The model under review builds one solid part; all positions refer to its coordinate system, in mm. Face numbers are marked on the shaded views. A direction names the side the tool comes from. Coordinates: 2 decimals unless noted, no trailing zeros. Write each loop counter-clockwise with the first axis right and the second up, starting at its lowest first coordinate (ties: lowest second). Pieces come first, ordered by that corner, then holes. Notation, with made-up numbers: (68, -33) - (85, -33) arc R14 ccw to (85, -19) - close; hole circle Ø7 at (-32, 88.5). An arc over 180 degrees is marked (long way). Put each result on its own line as item: value. Start each with the question number.
Item 1: Consider section A-A on y = 0. Give the boundary of the cut face in (x, z) (3 decimals).
Item 2: Consider section D-D on x = 4.5. Give the boundary of the cut face in (y, z).
Item 3: For pin 1 (10 mm diameter, centred on y = -10.5, z = 47.5, fed in from -X); pin 2 (10 mm diameter, centred on x = -6.5, z = 52.5, fed in from +Y); pin 3 (5.5 mm diameter, centred on x = 0, y = 0, fed in from +Z); pin 4 (8 mm diameter, centred on x = 4.5, z = 56, fed in from -Y), all flat-tipped, find the tip position at first contact; note any pin that passes through.
Item 4: Machinability: for the marked faces 1 and 2, which of the approach directions +Z, -Z, +X, -X, +Y, -Y give a long, thin tool a straight path to every point of the face, cutting with its end or side? Answer none if there is none.
Item 5: Consider section C-C on z = 33.5. Give the boundary of the cut face in (x, y) (3 decimals).
Item 6: To check wall thickness, follow L1, parallel to Y at x = 0, z = 19 (3 decimals); L2, parallel to Z at x = 10, y = -4; L3, parallel to X at y = -1, z = 7. State the ranges of each line that lie inside material, in increasing order. Write a range as [from, to].
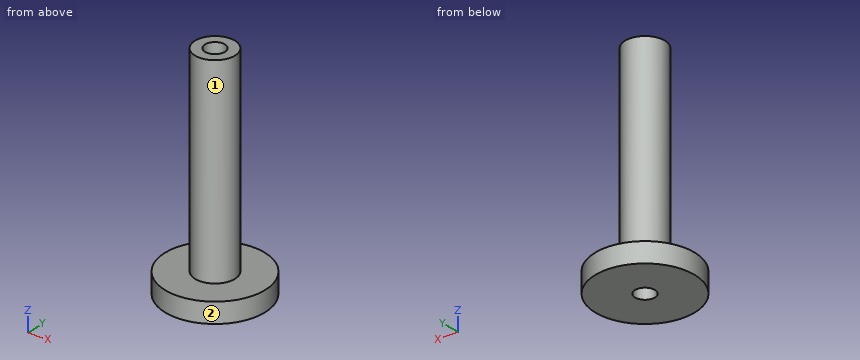
Autodesk Inventor part; units mm, degrees
ref_plane "YZ Plane" through (0, 0, 0) normal (1, 0, 0) x (0, 1, 0)
ref_plane "XZ Plane" through (0, 0, 0) normal (0, 1, 0) x (-1, 0, 0)
ref_plane "XY Plane" through (0, 0, 0) normal (0, 0, 1) x (1, 0, 0)
sketch "Sketch11" plane through (0, 0, 0) normal (0, 0, 1) x (1, 0, 0)
  circle A0 centre (0, 0) radius 15.875
  dimension "d21" = 31.75
extrude "Extrusion1" add sketch "Sketch11" along normal blind 6.35
sketch "Sketch12" plane through (0, 0, 6.35) normal (0, 0, 1) x (1, 0, 0)
  circle A0 centre (0, 0) radius 6.35
  dimension "d26" = 12.7
extrude "Extrusion2" add sketch "Sketch12" along normal blind 63.5
sketch "Sketch13" plane through (0, 0, 69.85) normal (0, 0, 1) x (1, 0, 0)
  circle A0 centre (0, 0) radius 3.175
  dimension "d27" = 6.35
extrude "Extrusion3" cut sketch "Sketch13" against normal through all
properties part number "punch_holder"
Report:
1. outline: (-15.875, 0) - (-3.175, 0) - (-3.175, 69.85) - (-6.35, 69.85) - (-6.35, 6.35) - (-15.875, 6.35) - close; (3.175, 0) - (15.875, 0) - (15.875, 6.35) - (6.35, 6.35) - (6.35, 69.85) - (3.175, 69.85) - close
2. outline: (-15.22, 0) - (15.22, 0) - (15.22, 6.35) - (4.48, 6.35) - (4.48, 69.85) - (-4.48, 69.85) - (-4.48, 6.35) - (-15.22, 6.35) - close
3. pin 1: x = -3.17
3. pin 2: y = 6.17
3. pin 3: through
3. pin 4: y = -6.33
4. face 1: +Z
4. face 2: +Z, -Z
5. outline: circle Ø12.7 at (0, 0); hole circle Ø6.35 at (0, 0)
6. L1: [-6.35, -3.175], [3.175, 6.35]
6. L2: [0, 6.35]
6. L3: [-6.27, -3.01], [3.01, 6.27]
